```python
from build123d import *

# Parameters (mm, degrees)
BOSS_EXTRUDE4_DEPTH           = 25
CUT_EXTRUDE2_DEPTH            = 25
TAP_DRILL_FOR_4_40_TAP1_D     = 1.600000102
TAP_DRILL_FOR_4_40_TAP1_DEPTH = 7.874
TAP_DRILL_FOR_4_40_TAP1_TIP   = 0.480688526
TAP_DRILL_FOR_4_40_TAP3_D     = 1.600000102
TAP_DRILL_FOR_4_40_TAP3_DEPTH = 7.874
TAP_DRILL_FOR_4_40_TAP3_TIP   = 0.480688526
TAP_DRILL_FOR_4_40_TAP4_D     = 1.600000102
TAP_DRILL_FOR_4_40_TAP4_DEPTH = 7.874
TAP_DRILL_FOR_4_40_TAP4_TIP   = 0.480688526
FILLET1_R                     = 1.778
CUT_EXTRUDE3_DEPTH            = 2.5
CUT_EXTRUDE4_DEPTH            = 2.5
CUT_EXTRUDE5_DEPTH            = 2.5
SKETCH23_W                    = 11
SKETCH23_H                    = 5.045
CUT_EXTRUDE6_DEPTH            = 5
SKETCH24_W                    = 11
SKETCH24_H                    = 5.045
CUT_EXTRUDE7_DEPTH            = 5
SKETCH25_W                    = 11
SKETCH25_H                    = 16.07506189
CUT_EXTRUDE8_DEPTH            = 10
SKETCH26_W                    = 184.458934752
SKETCH26_H                    = 50.4
BOSS_EXTRUDE6_DEPTH           = 29.21
SKETCH27_R                    = 3.429
CUT_EXTRUDE9_DEPTH            = 106.37252383
SKETCH28_W                    = 115.917353875
SKETCH28_H                    = 112.19052099
CUT_EXTRUDE10_DEPTH           = 119.151659651


with BuildPart() as part:
    # Sketch6 → Boss-Extrude4 (new body)
    with BuildSketch(Plane(origin=(0, 0, 0), x_dir=(1, 0, 0), z_dir=(0, 1, 0))):
        Polygon((-79.529467376, 0), (79.529467376, 0), (79.529467376, -56.321059428), (25, -63.5), (-25, -63.5), (-79.529467376, -56.321059428), align=None)
    extrude(amount=BOSS_EXTRUDE4_DEPTH)

    # Sketch7 → Cut-Extrude2 (cut, symmetric)
    with BuildSketch(Plane(origin=(0, 0, 0), x_dir=(0, 0, -1), z_dir=(1, 0, 0))):
        Polygon((-63.5, 25), (-38.5, 0), (-63.5, 0), align=None)
    extrude(amount=CUT_EXTRUDE2_DEPTH, both=True, mode=Mode.SUBTRACT)

    # Tap Drill for #4-40 Tap1
    with Locations(Plane(origin=(0, -19.25, 19.25), x_dir=(-1, 0, 0), z_dir=(0, -0.7071067811865488, 0.7071067811865462))):
        with Locations((-21.255000035, -53.756280605), (21.255000035, -53.756280605), (21.255000035, -36.046280605), (-21.255000035, -36.046280605)):
            Hole(TAP_DRILL_FOR_4_40_TAP1_D / 2, depth=TAP_DRILL_FOR_4_40_TAP1_DEPTH)
            with Locations((0, 0, -(TAP_DRILL_FOR_4_40_TAP1_DEPTH + TAP_DRILL_FOR_4_40_TAP1_TIP / 2))):  # 118° drill point
                Cone(0, TAP_DRILL_FOR_4_40_TAP1_D / 2, TAP_DRILL_FOR_4_40_TAP1_TIP, mode=Mode.SUBTRACT)

    # Tap Drill for #4-40 Tap3
    with Locations(Plane(origin=(-8.643431853, 0, 65.653383048), x_dir=(0.9914448613738104, 0, 0.13052619222005213), z_dir=(-0.13052619222005213, 0, 0.9914448613738104))):
        with Locations((-65.252708328, 21.355), (-22.742708328, 21.355), (-22.742708328, 3.645), (-65.252708328, 3.645)):
            Hole(TAP_DRILL_FOR_4_40_TAP3_D / 2, depth=TAP_DRILL_FOR_4_40_TAP3_DEPTH)
            with Locations((0, 0, -(TAP_DRILL_FOR_4_40_TAP3_DEPTH + TAP_DRILL_FOR_4_40_TAP3_TIP / 2))):  # 118° drill point
                Cone(0, TAP_DRILL_FOR_4_40_TAP3_D / 2, TAP_DRILL_FOR_4_40_TAP3_TIP, mode=Mode.SUBTRACT)

    # Tap Drill for #4-40 Tap4
    with Locations(Plane(origin=(8.643431853, 0, 65.653383048), x_dir=(0.9914448613738104, 0, -0.13052619222005213), z_dir=(0.13052619222005213, 0, 0.9914448613738104))):
        with Locations((22.742708328, 21.355), (65.252708328, 21.355), (65.252708328, 3.645), (22.742708328, 3.645)):
            Hole(TAP_DRILL_FOR_4_40_TAP4_D / 2, depth=TAP_DRILL_FOR_4_40_TAP4_DEPTH)
            with Locations((0, 0, -(TAP_DRILL_FOR_4_40_TAP4_DEPTH + TAP_DRILL_FOR_4_40_TAP4_TIP / 2))):  # 118° drill point
                Cone(0, TAP_DRILL_FOR_4_40_TAP4_D / 2, TAP_DRILL_FOR_4_40_TAP4_TIP, mode=Mode.SUBTRACT)

    # Fillet1
    fillet1_edges = [part.edges().sort_by_distance(p)[0] for p in [
        (-79.529467376, 25, 28.160529714),
        (79.529467376, 25, 28.160529714),
        (-79.529467376, 0, 28.160529714),
        (79.529467376, 0, 28.160529714),
    ]]
    fillet(fillet1_edges, radius=FILLET1_R)

    # Sketch22 → Cut-Extrude3 (cut)
    with BuildSketch(Plane(origin=(0, -19.25, 19.25), x_dir=(1, 0, 0), z_dir=(0, -0.7071067811865488, 0.7071067811865462))):
        Polygon((-19.055000086, 53.756280605), (-19.055000086, 50.756280605), (-22.055000086, 50.756280605), (-22.055000086, 39.046280605), (-19.055000086, 39.046280605), (-19.055000086, 36.046280605), (19.055000086, 36.046280605), (19.055000086, 39.046280605), (22.055000086, 39.046280605), (22.055000086, 50.756280605), (19.055000086, 50.756280605), (19.055000086, 53.756280605), align=None)
    extrude(amount=-CUT_EXTRUDE3_DEPTH, mode=Mode.SUBTRACT)

    # Sketch21 → Cut-Extrude4 (cut)
    with BuildSketch(Plane(origin=(8.643431853, 0, 65.653383048), x_dir=(0.9914448613738104, 0, -0.13052619222005213), z_dir=(0.13052619222005213, 0, 0.9914448613738104))):
        Polygon((24.942708277, 21.355), (24.942708277, 18.355), (21.942708277, 18.355), (21.942708277, 6.645), (24.942708277, 6.645), (24.942708277, 3.645), (63.052708379, 3.645), (63.052708379, 6.645), (66.052708379, 6.645), (66.052708379, 18.355), (63.052708379, 18.355), (63.052708379, 21.355), align=None)
    extrude(amount=-CUT_EXTRUDE4_DEPTH, mode=Mode.SUBTRACT)

    # Sketch20 → Cut-Extrude5 (cut)
    with BuildSketch(Plane(origin=(-8.643431853, 0, 65.653383048), x_dir=(0.9914448613738104, 0, 0.13052619222005213), z_dir=(-0.13052619222005213, 0, 0.9914448613738104))):
        Polygon((-63.052708379, 21.355), (-63.052708379, 18.355), (-66.052708379, 18.355), (-66.052708379, 6.645), (-63.052708379, 6.645), (-63.052708379, 3.645), (-24.942708277, 3.645), (-24.942708277, 6.645), (-21.942708277, 6.645), (-21.942708277, 18.355), (-24.942708277, 18.355), (-24.942708277, 21.355), align=None)
    extrude(amount=-CUT_EXTRUDE5_DEPTH, mode=Mode.SUBTRACT)

    # Sketch23 → Cut-Extrude6 (cut)
    with BuildSketch(Plane(origin=(8.643431853, 0, 65.653383048), x_dir=(0.9914448613738104, 0, -0.13052619222005213), z_dir=(0.13052619222005213, 0, 0.9914448613738104))):
        with Locations((43.997708328, 2.5225)):
            Rectangle(SKETCH23_W, SKETCH23_H)
    extrude(amount=-CUT_EXTRUDE6_DEPTH, mode=Mode.SUBTRACT)

    # Sketch24 → Cut-Extrude7 (cut)
    with BuildSketch(Plane(origin=(-8.643431853, 0, 65.653383048), x_dir=(0.9914448613738104, 0, 0.13052619222005213), z_dir=(-0.13052619222005213, 0, 0.9914448613738104))):
        with Locations((-43.997708328, 2.5225)):
            Rectangle(SKETCH24_W, SKETCH24_H)
    extrude(amount=-CUT_EXTRUDE7_DEPTH, mode=Mode.SUBTRACT)

    # Sketch25 → Cut-Extrude8 (cut)
    with BuildSketch(Plane(origin=(0, -19.25, 19.25), x_dir=(1, 0, 0), z_dir=(0, -0.7071067811865488, 0.7071067811865462))):
        with Locations((0, 29.40874966)):
            Rectangle(SKETCH25_W, SKETCH25_H)
    extrude(amount=-CUT_EXTRUDE8_DEPTH, mode=Mode.SUBTRACT)

    # Sketch26 → Boss-Extrude6 (add)
    with BuildSketch(Plane(origin=(0, 0, 0), x_dir=(-1, 0, 0), z_dir=(0, 0, -1))):
        with Locations((0, 12.5)):
            Rectangle(SKETCH26_W, SKETCH26_H)
    extrude(amount=-BOSS_EXTRUDE6_DEPTH)

    # Sketch11 → Cut-Revolve4 (revolve, cut)
    with BuildSketch(Plane(origin=(0, 0, 0), x_dir=(0, 0, -1), z_dir=(1, 0, 0))):
        with BuildLine():
            Line((1344.295, -496.77), (1344.295, 521.77))
            add(Edge.make_bspline(
                [(1344.295, 521.77), (-28.575, 521.77), (-28.575, 12.5), (-28.575, -496.77), (1344.295, -496.77)],
                knots=[4.71238898, 4.71238898, 4.71238898, 6.283185307, 6.283185307, 7.853981634, 7.853981634, 7.853981634], degree=2, weights=[1, 0.707106781, 1, 0.707106781, 1]))
        make_face()
    revolve(axis=Axis((0, -496.77, -1344.295), (0, 1, 0)), mode=Mode.SUBTRACT)

    # Sketch27 → Cut-Extrude9 (cut, through all)
    with BuildSketch(Plane.XY.offset(29.21)):
        with Locations((85.879467376, -6.35)):
            Circle(SKETCH27_R)
        with Locations((-85.879467376, -6.35)):
            Circle(SKETCH27_R)
        with Locations((-85.879467376, 31.35)):
            Circle(SKETCH27_R)
        with Locations((85.879467376, 31.35)):
            Circle(SKETCH27_R)
    extrude(amount=-CUT_EXTRUDE9_DEPTH, mode=Mode.SUBTRACT)

    # Sketch28 → Cut-Extrude10 (cut, through all)
    with BuildSketch(Plane(origin=(0, 0, 0), x_dir=(0, 0, -1), z_dir=(1, 0, 0))):
        with Locations((-70.629213931, -16.061676163)):
            Rectangle(SKETCH28_W, SKETCH28_H)
    extrude(amount=-CUT_EXTRUDE10_DEPTH, mode=Mode.SUBTRACT)


solid = part.part
```
Check sheet for the modelled part. Datum: model origin and axes. Units: mm. A direction names the side the tool comes from. Round coordinates to 2 decimals unless told otherwise and drop trailing zeros. Loops run counter-clockwise (first coordinate to the right, second up) from the corner with the lowest first, then second, coordinate; pieces in that order, holes last. Notation, with made-up numbers: (62, 26) -> (82, 26) arc R30 cw to (82, 50) -> close; hole circle Ø2 at (60.25, -30). An arc over 180 degrees is marked (long way). Answer in a Markdown table with one row per item.
Q1. Go/stop test with flat-tipped pins: P1, Ø10, axis at x = 15.5, y = 8.5, coming from the -Z side; P2, Ø5, axis at y = 0.5, z = 29.5, coming from the +X side; P3, Ø10, axis at x = 16.5, y = 8.5, coming from the +Z side; P4, Ø2.5, axis at x = 72, z = 56.5, coming from the -Y side. Record where each tip stops, or that it passes through.
Data:
| item | result |
|---|---|
| P1 | stops at z = 28.27 |
| P2 | stops at x = 92.23 |
| P3 | stops at z = 48.46 |
| P4 | stops at y = 0 |
Q2. Thickness scan on L1, parallel to X at y = 21, z = 46; L2, parallel to Y at x = 51.5, z = 46; L3, parallel to X at y = -4, z = 28. Record the ranges inside material, lowest first.
Data:
| item | result |
|---|---|
| L1 | x = 0 to 79.53 |
| L2 | y = 0 to 25 |
| L3 | x = 0 to 83.38, 88.38 to 92.23 |
Q3. Set-up check for faces 1 (the face through (79.529, 12, 43)), 2 (the face through (39, 25, 46)), 3 (the face through (20.53, 9.23, 45.99)), 4 (the face through (48, 0, 42)), 5 (the face through (19.055, 19, 55)): record each of +Z, -Z, +X, -X, +Y, -Y from which the full face is reachable in a straight line by a thin tool's end or side.
Data:
| item | result |
|---|---|
| face 1 | +Z, +X, +Y, -Y |
| face 2 | +Z, +X, -X, +Y |
| face 3 | +Z, -X |
| face 4 | +Z, +X, -X, -Y |
| face 5 | -X, -Y |
Q4. Sectioned sample at A-A on z = 35.5. Enter the section's corners in (x, y), then the cut area to 3 significant figures.
Data:
| item | result |
|---|---|
| outline | (0, 11.14) -> (5.5, 11.14) -> (5.5, 0) -> (77.75, 0) arc R1.78 ccw to (79.53, 1.78) -> (79.53, 23.22) arc R1.78 ccw to (77.75, 25) -> (0, 25) -> close |
| area | 1,930 mm^2 |
Q5. Release check for a two-part mould opening along Z. For faces 6 (the face through (52.65, 23.44, 59.86)), 7 (the face through (92.229, 12, 27)), 8 (the face through (33.212, 19.876, 61.176)) record: released by +Z, released by -Z, zero draft, split by the parting line, or undercut.
Data:
| item | result |
|---|---|
| face 6 | released by +Z |
| face 7 | zero draft |
| face 8 | undercut |
